from build123d import *

# Parameters (mm, degrees)
SKETCH1_W               = 195.58
SKETCH1_H               = 38.1
BOSS_EXTRUDE1_DEPTH     = 19.05
SKETCH2_R               = 12.8984375
CUT_EXTRUDE1_DEPTH      = 20.05
CUT_EXTRUDE2_DEPTH      = 20.05
SKETCH4_W               = 19.05
SKETCH4_H               = 19.05
BOSS_EXTRUDE2_DEPTH     = 50.8
SKETCH6_R               = 3.302
CUT_EXTRUDE3_DEPTH      = 196.58
FILLET1_R               = 6.35
FILLET2_R               = 1.5875
SKETCH7_W               = 86.796683621
SKETCH7_H               = 6.35
BOSS_EXTRUDE3_DEPTH     = 19.05
SKETCH8_W               = 30.563761808
SKETCH8_H               = 20.145620364
CUT_EXTRUDE4_DEPTH      = 1
CUT_EXTRUDE4_DEPTH_BACK = 20.05


with BuildPart() as part:
    # Sketch1 → Boss-Extrude1 (new body)
    with BuildSketch(Plane.XY):
        Rectangle(SKETCH1_W, SKETCH1_H)
    extrude(amount=BOSS_EXTRUDE1_DEPTH)

    # Sketch2 → Cut-Extrude1 (cut, through all)
    with BuildSketch(Plane.XY.offset(19.05)):
        with Locations((-56.515, 0)):
            Circle(SKETCH2_R)
        with Locations((56.515, 0)):
            Circle(SKETCH2_R)
    extrude(amount=-CUT_EXTRUDE1_DEPTH, mode=Mode.SUBTRACT)

    # Sketch3 → Cut-Extrude2 (cut, through all)
    with BuildSketch(Plane.XY.offset(19.05)):
        with BuildLine():
            Line((-15.281880904, -5.254379636), (-10.086091047, -21.968397565))
            Line((-10.086091047, -21.968397565), (10.086091047, -21.968397565))
            Line((10.086091047, -21.968397565), (15.281880904, -5.254379636))
            ThreePointArc((15.281880904, -5.254379636), (0, 15.493999988), (-15.281880904, -5.254379636))
        make_face()
    extrude(amount=-CUT_EXTRUDE2_DEPTH, mode=Mode.SUBTRACT)

    # Sketch4 → Boss-Extrude2 (add)
    with BuildSketch(Plane.ZY.offset(97.79)):
        with Locations((9.525, 28.575)):
            Rectangle(SKETCH4_W, SKETCH4_H)
    boss_extrude2 = extrude(amount=-BOSS_EXTRUDE2_DEPTH)

    # Sketch6 → Cut-Extrude3 (cut, through all)
    with BuildSketch(Plane.ZY.offset(97.79)):
        with Locations((9.525, 31.75)):
            Circle(SKETCH6_R)
    cut_extrude3 = extrude(amount=-CUT_EXTRUDE3_DEPTH, mode=Mode.SUBTRACT)

    # Mirror2: Boss-Extrude2, Cut-Extrude3 across plane
    add(boss_extrude2.mirror(Plane(origin=(0, 0, 0), x_dir=(0, 0, 1), z_dir=(1, 0, 0))))
    add(cut_extrude3.mirror(Plane(origin=(0, 0, 0), x_dir=(0, 0, 1), z_dir=(1, 0, 0))), mode=Mode.SUBTRACT)

    # Fillet1
    fillet1_edges = [part.edges().sort_by_distance(p)[0] for p in [
        (-46.99, 19.05, 9.525),
        (46.99, 19.05, 9.525),
    ]]
    fillet(fillet1_edges, radius=FILLET1_R)

    # Fillet2
    fillet2_edges = [part.edges().sort_by_distance(p)[0] for p in [
        (-46.99, 38.1, 9.525),
        (-97.79, 38.1, 9.525),
        (97.79, 38.1, 9.525),
        (46.99, 38.1, 9.525),
    ]]
    fillet(fillet2_edges, radius=FILLET2_R)

    # Sketch7 → Boss-Extrude3 (add)
    with BuildSketch(Plane.XY.offset(19.05)):
        with Locations((-54.39165819, -22.225)):
            Rectangle(SKETCH7_W, SKETCH7_H)
        with Locations((54.39165819, -22.225)):
            Rectangle(SKETCH7_W, SKETCH7_H)
    extrude(amount=-BOSS_EXTRUDE3_DEPTH)

    # Sketch8 → Cut-Extrude4 (cut, two sides)
    with BuildSketch(Plane.XY.offset(19.05)) as cut_extrude4_sk:
        with Locations((0, -15.327189818)):
            Rectangle(SKETCH8_W, SKETCH8_H)
    extrude(amount=CUT_EXTRUDE4_DEPTH, mode=Mode.SUBTRACT)
    extrude(cut_extrude4_sk.sketch, amount=-CUT_EXTRUDE4_DEPTH_BACK, mode=Mode.SUBTRACT)


solid = part.part
Build history of the part. All positions in model axes, mm. A direction names the side the tool comes from. Round coordinates to 2 decimals unless told otherwise and drop trailing zeros. Write each loop counter-clockwise with the first axis right and the second up, starting at its lowest first coordinate (ties: lowest second). Pieces come first, ordered by that corner, then holes. Notation, with made-up numbers: M 26,47.5 L 38,47.5 A25 ccw 38,66.5 Z; hole C 2,-20.5 d3. An arc over 180 degrees is marked long. Answer in a Markdown table with one row per item.
1. Saw through at A-A (y = 11). List the corners of the cut face in (x, z), and give its area (3 significant figures).
Geometry check:
| item | result |
|---|---|
| outline | M -97.79,0 L -63.25,0 L -63.25,19.05 L -97.79,19.05 Z; M -49.78,0 L -11.12,0 L -11.12,19.05 L -49.78,19.05 Z; M 11.12,0 L 49.78,0 L 49.78,19.05 L 11.12,19.05 Z; M 63.25,0 L 97.79,0 L 97.79,19.05 L 63.25,19.05 Z |
| area | 2,790 mm2 |
2. Which spindle directions (+Z, -Z, +X, -X, +Y, -Y) get a long thin tool onto all of the face, cutting with end or side? Do faces 4 (the face through (-1, 19.05, 9)), 5 (the face through (15.282, -15, 10)), 6 (the face through (-57, -25.4, 10)). Say none if no direction does.
Geometry check:
| item | result |
|---|---|
| face 4 | +Z, -Z, +Y |
| face 5 | +Z, -Z, -Y |
| face 6 | +Z, -Z, +X, -X, -Y |
3. Saw through at C-C (x = 62.5). List the corners of the cut face in (y, z) (3 decimals).
Geometry check:
| item | result |
|---|---|
| outline | M -25.4,0 L -11.426,0 L -11.426,19.05 L -25.4,19.05 Z; M 11.426,0 L 38.1,0 L 38.1,19.05 L 11.426,19.05 Z; hole C 31.75,9.525 d6.604 |
4. Saw through at D-D (y = 31.75). List the corners of the cut face in (x, z), and give its area (3 significant figures).
Geometry check:
| item | result |
|---|---|
| outline | M -97.79,0 L -46.99,0 L -46.99,6.22 L -97.79,6.22 Z; M -97.79,12.83 L -46.99,12.83 L -46.99,19.05 L -97.79,19.05 Z; M 46.99,0 L 97.79,0 L 97.79,6.22 L 46.99,6.22 Z; M 46.99,12.83 L 97.79,12.83 L 97.79,19.05 L 46.99,19.05 Z |
| area | 1,260 mm2 |
5. Mould opens along Z. For faces 1 (the face through (-15.282, -15, 10)), 2 (the face through (-72.746, 28.527, 8.809)), 3 (the face through (20, 0, 0)) say: +Z half, -Z half, draft (parallel to the pull), parting line (faces both ways), or undercut.
Geometry check:
| item | result |
|---|---|
| face 1 | draft |
| face 2 | undercut |
| face 3 | -Z half |
6. Saw through at B-B (z = 15.25). State how many separate pieces and enclosed holes the cut face has, and give its area (3 significant figures).
Geometry check:
| item | result |
|---|---|
| separate pieces | 1 |
| enclosed holes | 2 |
| area | 8,430 mm2 |
7. Flat gauge pin, fed straight in: P1, Ø10, axis at x = -11.5, z = 16.5, coming from the +Y side. Where does the tip first touch, or does it go through?
Geometry check:
| item | result |
|---|---|
| P1 | y = 19.05 |
8. Probe L1, parallel to Y at x = -70.5, z = 10; L2, parallel to X at y = -6.5, z = 5; L3, parallel to X at y = 7.5, z = 3.5. List the from-to ranges inside material, lowest first. Write a range as [from, to].
Geometry check:
| item | result |
|---|---|
| L1 | [-25.4, 28.48], [35.02, 38.1] |
| L2 | [-97.79, -67.66], [-45.37, -15.28], [15.28, 45.37], [67.66, 97.79] |
| L3 | [-97.79, -67.01], [-46.02, -13.85], [13.85, 46.02], [67.01, 97.79] |
